For this review, take the finished solid that the model builds, in its own axes (mm). A direction names the side the tool comes from. Round coordinates to 2 decimals unless told otherwise and drop trailing zeros. Loops run counter-clockwise (first coordinate to the right, second up) from the corner with the lowest first, then second, coordinate; pieces in that order, holes last.
```python
from build123d import *

# Parameters (mm, degrees)
BOSS_EXTRUDE1_DEPTH    = 6.35
F_10_CLEARANCE_HOLE1_D = 5.1054
CUT_EXTRUDE1_REACH     = 69.651
SKETCH4_R              = 2.38125
CHAMFER1_SIZE          = 1.27


with BuildPart() as part:
    # Sketch1 → Boss-Extrude1 (new, symmetric)
    with BuildSketch(Plane(origin=(0, 0, 0), x_dir=(0, 0, -1), z_dir=(1, 0, 0))):
        Polygon((0, 0), (31.75, 0), (31.75, 2.794), (66.675, 2.794), (66.675, 9.525), (0, 9.525), align=None)
    extrude(amount=BOSS_EXTRUDE1_DEPTH, both=True)

    # #10 Clearance Hole1 (through all)
    with Locations(Plane(origin=(0, 0, 0), x_dir=(-1, 0, 0), z_dir=(0, -1, 0))):
        with Locations((0, 23.65375), (0, 10.95375)):
            Hole(F_10_CLEARANCE_HOLE1_D / 2)

    # Sketch4 → Cut-Extrude1 (cut, up to next)
    with BuildSketch(Plane(origin=(0, 9.525, 0), x_dir=(1, 0, 0), z_dir=(0, 1, 0)), mode=Mode.PRIVATE) as cut_extrude1_sk1:
        with Locations(Location((0, 61.75375, 0), (0, 0, 270))):
            Circle(SKETCH4_R)
    cut_extrude1_tool1 = extrude(cut_extrude1_sk1.sketch, amount=-CUT_EXTRUDE1_REACH, mode=Mode.PRIVATE) & part.part
    add(cut_extrude1_tool1.solids().sort_by_distance((0, 9.525, -61.75375))[0], mode=Mode.SUBTRACT)

    # Chamfer1
    chamfer1_edges = [part.edges().sort_by_distance(p)[0] for p in [
        (0, 2.794, -66.675),
    ]]
    chamfer(chamfer1_edges, length=CHAMFER1_SIZE)


solid = part.part
```
(1) Insertion check: pin 1 Ø0.8 at (x, y) = (3, 2) entering from -Z. The pin has a flat end and moves straight along its axis. Give the tip position at first contact, or say it passes through.
(2) Add section A-A (x = 0). Give the number of separate pieces and of enclosed holes in the cut face, plus the area to 3 significant figures.
(3) Add section B-B (x = 4). Give the boundary of the cut face in (y, z) (3 decimals).
(4) Add section D-D (y = 1). Give the boundary of the cut face in (x, z), plus the area to 3 significant figures.
(5) For faces 1 (the flat face through (-6.35, 6, -33)), 2 (the flat face through (0, 2.794, -48)), list the 3-axis set-ups (+Z, -Z, +X, -X, +Y, -Y) from which the entire face can be reached by the end or side of a thin tool; tool diameter is ignored.
(6) For L1, parallel to X at y = 0.5, z = -11; L2, parallel to Z at x = -0.75, y = 4.25 (3 decimals); L3, parallel to Z at x = -2.75, y = 2, list the stretches that pass through material, from the lowest coordinate up.
(7) The part is to be moulded in two halves that separate along X. For faces 3 (the flat face through (0, 7, -66.675)), 4 (the cylindrical face through (-0.55, 4.83, -8.46)), 5 (the cylindrical face through (0.105, 6.207, -64.133)), 6 (the flat face through (6.35, 6, -33)), say which applies: pulls with the +X half, pulls with the -X half, needs draft (parallel to the pull), parting line crosses it, or undercut.
Outcome:
1. pin 1: stops at z = -31.75
2. separate pieces: 4
2. enclosed holes: 0
2. area: 407 mm2
3. outline: (0, -31.75) - (2.794, -31.75) - (2.794, -65.405) - (4.064, -66.675) - (9.525, -66.675) - (9.525, 0) - (0, 0) - close
4. outline: (-6.35, -31.75) - (6.35, -31.75) - (6.35, 0) - (-6.35, 0) - close; hole circle Ø5.11 at (0, -23.65); hole circle Ø5.11 at (0, -10.95)
4. area: 362 mm2
5. face 1: +Z, -Z, -X, +Y, -Y
5. face 2: -Z, +X, -X, -Y
6. L1: x = -6.35 to -2.55, 2.55 to 6.35
6. L2: z = -66.675 to -64.014, -59.494 to -26.094, -21.214 to -13.394, -8.514 to 0
6. L3: z = -31.75 to 0
7. face 3: needs draft
7. face 4: undercut
7. face 5: undercut
7. face 6: pulls with the +X half
